Could you check a few things on this model? Use its own coordinates, in mm. Face numbers are marked on the shaded views. A direction names the side the tool comes from. Round coordinates to 2 decimals unless told otherwise and drop trailing zeros. Loops run counter-clockwise (first coordinate to the right, second up) from the corner with the lowest first, then second, coordinate; pieces in that order, holes last. Notation, with made-up numbers: (85.5, -7.75) -> (128.5, -7.75) arc R30 ccw to (128.5, 21.25) -> close; hole circle Ø7 at (10, 17). An arc over 180 degrees is marked (long way). Put each result on its own line as item: value. Start each with the question number.
1. Which directions (+Z, -Z, +X, -X, +Y, -Y) give clear straight access to the entire face, cutting with the end or side of a thin tool? Please do the marked faces 5 and 6.
2. Imagine slicing it at A-A, the plane z = 9.5. Please give me the cut outline in (x, y).
3. If we mould it in two halves opening along Y, with no side actions, what happens to the marked faces 1, 2, 3 and 4? For each: pulls with the +Y half, pulls with the -Y half, needs draft (parallel to the pull), parting line crosses it, or undercut.
4. I'm going to push flat-ended pins straight in: P1, Ø2, axis at x = -11, z = 5.5, coming from the +Y side; P2, Ø0.5, axis at x = 16.5, z = 2.5, coming from the -Y side; P3, Ø0.8, axis at y = 49.5, z = 0.5, coming from the +X side. Where does each tip first touch, or does it pass through?
5. Imagine slicing it at D-D, the plane y = -13. Please give me the cut outline in (x, z), and give its area (3 significant figures).
6. Imagine slicing it at C-C, the plane x = -10. Please give me the cut outline in (y, z).
7. Imagine slicing it at B-B, the plane x = 8.5. Please give me the cut outline in (y, z).
8. I need wall thicknesses on line 1 (Y direction, x = -18, z = 4.25); line 2 (Y direction, x = 4.5, z = 10); line 3 (Y direction, x = -4.5, z = 4.5). Which ranges of each line are inside material? Lowest first, please. Write a range as [from, to].
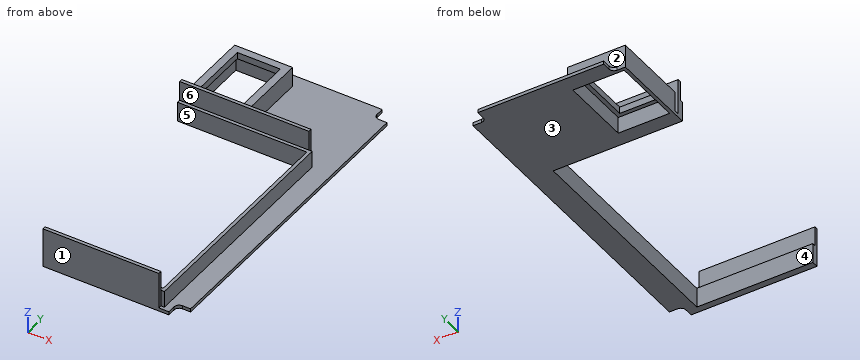
```python
from build123d import *

# Parameters (mm, degrees)
F2_W      = 46
F2_H      = 101
F3_DEPTH  = 1
F5_DEPTH  = 1
F6_W      = 39
F6_H      = 68
F7_DEPTH  = 1
F8_W      = 39
F8_H      = 1
F8_W_2    = 35
F9_DEPTH  = 11
F10_W     = 1
F10_H     = 68
F11_DEPTH = 5
F12_W     = 17.5
F12_H     = 23.5
F12_W_2   = 15.5
F12_H_2   = 21.5
F13_DEPTH = 4
F14_W     = 15.5
F14_H     = 21.5
F15_DEPTH = 1
F16_W     = 17.5
F16_H     = 23.5
F16_W_2   = 13
F16_H_2   = 19
F17_DEPTH = 2


with BuildPart() as f3:
    # F2 (on Top) → F3 (new body)
    with BuildSketch(Plane.XY):
        Rectangle(F2_W, F2_H)
    extrude(amount=F3_DEPTH)

    # F4 (on face) → F5 (cut, through all)
    with BuildSketch(Plane.XY.offset(1)):
        with BuildLine():
            Line((-19, 50.5), (-23, 50.5))
            Line((-23, 50.5), (-23, 46.5))
            Line((-23, 46.5), (-20.5, 46.5))
            ThreePointArc((-20.5, 46.5), (-19.4393398282, 46.9393398282), (-19, 48))
            Line((-19, 48), (-19, 50.5))
        make_face()
        with BuildLine():
            Line((23, 46.5), (23, 50.5))
            Line((23, 50.5), (19, 50.5))
            Line((19, 50.5), (19, 48))
            ThreePointArc((19, 48), (19.4393398282, 46.9393398282), (20.5, 46.5))
            Line((20.5, 46.5), (23, 46.5))
        make_face()
        with BuildLine():
            Line((23, -46.5), (20.5, -46.5))
            ThreePointArc((20.5, -46.5), (19.4393398282, -46.9393398282), (19, -48))
            Line((19, -48), (19, -50.5))
            Line((19, -50.5), (23, -50.5))
            Line((23, -50.5), (23, -46.5))
        make_face()
        with BuildLine():
            ThreePointArc((-19, -48), (-19.4393398282, -46.9393398282), (-20.5, -46.5))
            Line((-20.5, -46.5), (-23, -46.5))
            Line((-23, -46.5), (-23, -50.5))
            Line((-23, -50.5), (-19, -50.5))
            Line((-19, -50.5), (-19, -48))
        make_face()
    extrude(amount=-F5_DEPTH, mode=Mode.SUBTRACT)

    # F6 (on face) → F7 (cut, through all)
    with BuildSketch(Plane.XY.offset(1)):
        with Locations((-3.5, -14.5)):
            Rectangle(F6_W, F6_H)
    extrude(amount=-F7_DEPTH, mode=Mode.SUBTRACT)

    # F8 (on face) → F9 (join)
    with BuildSketch(Plane.XY.offset(1)):
        with Locations((-3.5, 21)):
            Rectangle(F8_W, F8_H)
        with Locations((-1.5, -50)):
            Rectangle(F8_W_2, F8_H)
    extrude(amount=F9_DEPTH)

    # F10 (on face) → F11 (join)
    with BuildSketch(Plane.XY.offset(1)):
        Polygon((-23, 20.5), (-23, 19.5), (16, 19.5), (17, 19.5), (17, 20.5), align=None)
        with Locations((16.5, -14.5)):
            Rectangle(F10_W, F10_H)
        Polygon((17, -48.5), (16, -48.5), (-19, -48.5), (-19, -49.5), (17, -49.5), align=None)
    extrude(amount=F11_DEPTH)

    # F12 (on face) → F13 (join)
    with BuildSketch(Plane.XY.offset(1)):
        with Locations((-14.25, 34.75)):
            Rectangle(F12_W, F12_H)
        with Locations((-14.25, 34.75)):
            Rectangle(F12_W_2, F12_H_2, mode=Mode.SUBTRACT)
    extrude(amount=F13_DEPTH)

    # F14 (on face) → F15 (cut, through all)
    with BuildSketch(Plane.XY.offset(1)):
        with Locations((-14.25, 34.75)):
            Rectangle(F14_W, F14_H)
    extrude(amount=-F15_DEPTH, mode=Mode.SUBTRACT)

    # F16 (on face) → F17 (join)
    with BuildSketch(Plane.XY.offset(5)):
        with Locations((-14.25, 34.75)):
            Rectangle(F16_W, F16_H)
        with Locations((-14.25, 34.75)):
            Rectangle(F16_W_2, F16_H_2, mode=Mode.SUBTRACT)
    extrude(amount=F17_DEPTH)


solid = f3.part
```
Entries:
1. face 5: +Z, -Z, -X
1. face 6: +Z, +X, -X
2. outline: (-23, 20.5) -> (16, 20.5) -> (16, 21.5) -> (-23, 21.5) -> close; (-19, -50.5) -> (16, -50.5) -> (16, -49.5) -> (-19, -49.5) -> close
3. face 1: pulls with the -Y half
3. face 2: pulls with the +Y half
3. face 3: needs draft
3. face 4: undercut
4. P1: y = 46.5
4. P2: y = -49.5
4. P3: x = 19
5. outline: (16, 0) -> (23, 0) -> (23, 1) -> (17, 1) -> (17, 6) -> (16, 6) -> close
5. area: 12.0 mm^2
6. outline: (-50.5, 0) -> (-48.5, 0) -> (-48.5, 6) -> (-49.5, 6) -> (-49.5, 12) -> (-50.5, 12) -> close; (19.5, 0) -> (24, 0) -> (24, 5) -> (25.25, 5) -> (25.25, 7) -> (23, 7) -> (23, 1) -> (21.5, 1) -> (21.5, 12) -> (20.5, 12) -> (20.5, 6) -> (19.5, 6) -> close; (44.25, 5) -> (45.5, 5) -> (45.5, 0) -> (50.5, 0) -> (50.5, 1) -> (46.5, 1) -> (46.5, 7) -> (44.25, 7) -> close
7. outline: (-50.5, 0) -> (-48.5, 0) -> (-48.5, 6) -> (-49.5, 6) -> (-49.5, 12) -> (-50.5, 12) -> close; (19.5, 0) -> (50.5, 0) -> (50.5, 1) -> (21.5, 1) -> (21.5, 12) -> (20.5, 12) -> (20.5, 6) -> (19.5, 6) -> close
8. line 1: [-50.5, -48.5], [19.5, 21.5], [23, 24], [45.5, 46.5]
8. line 2: [-50.5, -49.5], [20.5, 21.5]
8. line 3: [-50.5, -48.5], [19.5, 21.5]
